Build history of the part. All positions in model axes, mm. Face numbers are marked on the shaded views. Round coordinates to 2 decimals unless told otherwise and drop trailing zeros. Loops run counter-clockwise (first coordinate to the right, second up) from the corner with the lowest first, then second, coordinate; pieces in that order, holes last. Notation, with made-up numbers: (86.25, -4.5) - (95.25, -4.5) arc R19 ccw to (95.25, 5.5) - close; hole circle Ø8 at (-31, -7). An arc over 180 degrees is marked (long way). Use a Markdown table: item, result.
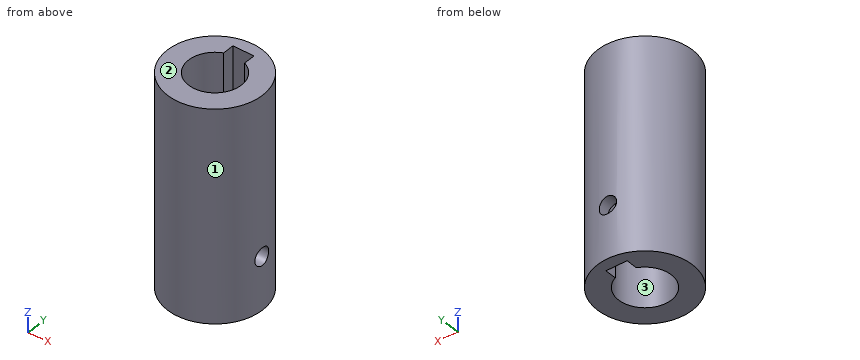
from build123d import *

# Parameters (mm, degrees)
SKETCH_1_R               = 9
SKETCH_1_R_2             = 5
EXTRUDE_1_DEPTH          = 40
SKETCH_2_W               = 4
SKETCH_2_H               = 3.302981626
CUT_EXTRUDE_2_DEPTH      = 42.976183724
SKETCH_3_W               = 1.65
SKETCH_3_H               = 9
PATTERN_CIRCULAR_1_COUNT = 2
PATTERN_CIRCULAR_1_ANGLE = 90


with BuildPart() as part:
    # 草图1 → 拉伸1 (new body)
    with BuildSketch(Plane.XY):
        Circle(SKETCH_1_R)
        Circle(SKETCH_1_R_2, mode=Mode.SUBTRACT)
    extrude(amount=EXTRUDE_1_DEPTH)

    # 草图2 → 拉伸2 (cut, through all)
    with BuildSketch(Plane.XY.offset(40)):
        with Locations((0, 5.148509187)):
            Rectangle(SKETCH_2_W, SKETCH_2_H)
    extrude(amount=-CUT_EXTRUDE_2_DEPTH, mode=Mode.SUBTRACT)

    # 草图3 → M4 螺纹孔2 (revolve, cut)
    with BuildSketch(Plane(origin=(0, 0, 10), x_dir=(0, 0, -1), z_dir=(1, 0, 0))):
        with Locations((0.825, 4.5)):
            Rectangle(SKETCH_3_W, SKETCH_3_H)
    hole_wizard_m4_2 = revolve(axis=Axis((0, -6.35, 10), (0, 1, 0)), mode=Mode.SUBTRACT)

    # 阵列(圆周)1: M4 螺纹孔2 ×2 about axis
    pattern_circular_1_axis = Axis((0, 0, 40), (0, 0, -1))
    for i in range(1, PATTERN_CIRCULAR_1_COUNT):
        add(hole_wizard_m4_2.rotate(pattern_circular_1_axis, i * PATTERN_CIRCULAR_1_ANGLE / (PATTERN_CIRCULAR_1_COUNT - 1)), mode=Mode.SUBTRACT)


solid = part.part
Q1. Probe line 1 (Y direction, x = 0, z = 3.5); line 2 (Z direction, x = 0, y = 8.4); line 3 (X direction, y = 0.25, z = 35). List the from-to ranges inside material, lowest first.
Results found:
| item | result |
|---|---|
| line 1 | y = -9 to -5, 6.8 to 9 |
| line 2 | z = 0 to 8.35, 11.65 to 40 |
| line 3 | x = -9 to -4.99, 4.99 to 9 |
Q2. Pull direction X, two halves, no side cores. Call the marked faces 1, 2 and 3: pulls with the +X half, pulls with the -X half, needs draft (parallel to the pull), parting line crosses it, or undercut.
Results found:
| item | result |
|---|---|
| face 1 | parting line crosses it |
| face 2 | needs draft |
| face 3 | undercut |
Q3. Cut at D-D, the plane z = 32. List the corners of the cut face in (x, y), plus the area to 3 significant figures.
Results found:
| item | result |
|---|---|
| outline | circle Ø18 at (0, 0); hole (-2, 4.58) arc R5 ccw (long way) to (2, 4.58) - (2, 6.8) - (-2, 6.8) - close |
| area | 168 mm2 |
Q4. Cut at C-C, the plane x = -4. List the corners of the cut face in (y, z), plus the area to 3 significant figures.
Results found:
| item | result |
|---|---|
| outline | (-8.06, 0) - (-3, 0) - (-3, 40) - (-8.06, 40) - close; (3, 0) - (8.06, 0) - (8.06, 40) - (3, 40) - close |
| area | 405 mm2 |
Q5. Drop flat-ended pins along their axis: pin 1 (2.5 mm diameter, centred on y = 6, z = 15, fed in from +X); pin 2 (2 mm diameter, centred on y = 0, z = 10, fed in from +X); pin 3 (6 mm diameter, centred on x = 6, z = 31, fed in from -Y). Give the stop position or say it passes through.
Results found:
| item | result |
|---|---|
| pin 1 | stops at x = 7.64 |
| pin 2 | stops at x = -4.9 |
| pin 3 | stops at y = -8.49 |
Q6. Cut at A-A, the plane y = 0. List the corners of the cut face in (x, z).
Results found:
| item | result |
|---|---|
| outline | (-9, 0) - (-5, 0) - (-5, 40) - (-9, 40) - close; (5, 0) - (9, 0) - (9, 8.35) - (5, 8.35) - close; (5, 11.65) - (9, 11.65) - (9, 40) - (5, 40) - close |
Q7. Cut at B-B, the plane x = 0. List the corners of the cut face in (y, z).
Results found:
| item | result |
|---|---|
| outline | (-9, 0) - (-5, 0) - (-5, 40) - (-9, 40) - close; (6.8, 0) - (9, 0) - (9, 8.35) - (6.8, 8.35) - close; (6.8, 11.65) - (9, 11.65) - (9, 40) - (6.8, 40) - close |
